from build123d import *

# Parameters (mm, degrees)
F0_R     = 4.7625
F1_DEPTH = 117.856
F2_W     = 9.525
F2_H     = 32.258
F3_DEPTH = 25.4
F4_DEPTH = 0.6985
F5_R     = 1.778
F6_DEPTH = 25.4
F8_DEPTH = 6.35
F9_SIZE  = 0.635


with BuildPart() as f1:
    # F0 (on Top) → F1 (new body)
    with BuildSketch(Plane.XY):
        Circle(F0_R)
    extrude(amount=F1_DEPTH)

    # F2 (on Right) → F3 (cut)
    with BuildSketch(Plane.YZ):
        with Locations((0, 29.337)):
            Rectangle(F2_W, F2_H)
    extrude(amount=F3_DEPTH, mode=Mode.SUBTRACT)

    # F2 (on Right) → F4 (cut)
    with BuildSketch(Plane.YZ):
        with Locations((0, 29.337)):
            Rectangle(F2_W, F2_H)
    extrude(amount=-F4_DEPTH, mode=Mode.SUBTRACT)

    # F5 (on face) → F6 (cut)
    with BuildSketch(Plane.YZ):
        with Locations((0, 39.6748)):
            Circle(F5_R)
        with Locations((0, 18.9738)):
            Circle(F5_R)
    extrude(amount=-F6_DEPTH, mode=Mode.SUBTRACT)

    # F7 (on face) → F8 (join)
    with BuildSketch(Plane.XY):
        with BuildLine():
            Line((3.928686, -2.691995), (3.928686, 2.691995))
            ThreePointArc((3.928686, 2.691995), (-4.7625, 0), (3.928686, -2.691995))
        make_face()
    extrude(amount=-F8_DEPTH)

    # F9
    f9_edges = [f1.edges().sort_by_distance(p)[0] for p in [
        (-4.7625, 0, 117.856),
    ]]
    chamfer(f9_edges, length=F9_SIZE)


solid = f1.part
Geometry: final body of the model. Coordinates: model frame, mm. A direction names the side the tool comes from. Give positions to 0.01 mm unless a question says otherwise; leave off trailing zeros. Write each loop counter-clockwise with the first axis right and the second up, starting at its lowest first coordinate (ties: lowest second). Pieces come first, ordered by that corner, then holes. Notation, with made-up numbers: (72, 79) - (110, 79) arc R27 cw to (110, 108) - close; hole circle Ø10 at (4, 36). An arc over 180 degrees is marked (long way). Return JSON: item names as keys, results as strings. Group by question number.
1) Set-up query: faces 3 (the flat face through (3.929, 0, -3)), 4 (the flat face through (-0.698, 0, 30)), 5 (the flat face through (0, 0, -6.35)). Return all of +Z, -Z, +X, -X, +Y, -Y with unobstructed straight access to the full face (end or side cutting, diameter ignored); none if empty.
2) Section B-B on z = 25.5. Return the cut outline in (x, y) (1 decimal).
3) Mould query, pull axis Y, two halves, no side actions, for faces 1 (the cylindrical face through (-2.703, -1.776, 39.753)), 2 (the flat face through (0, 0, 117.856)). Classes: released by +Y, released by -Y, zero draft, split by the parting line, or undercut.
4) Section A-A on y = 0. Return the cut outline in (x, z).
5) First-contact query: P1, Ø1, axis at y = -2.5, z = 94, coming from the -X side; P2, Ø5.5, axis at y = 0, z = 39.67, coming from the +X side; P3, Ø2, axis at y = -2, z = 39, coming from the -X side. Flat tips, straight axial feed; report the tip coordinate or a pass-through.
6) Section D-D on z = 103. Return the cut outline in (x, y) (1 decimal), plus the area to 3 significant figures.
7) Section C-C on x = -1.75. State how many separate pieces and enclosed holes the cut face has, plus the area to 3 significant figures.
8) Line query: line 1 (Z direction, x = -2.25, y = 0); line 2 (Z direction, x = 0, y = 2.75); line 3 (Y direction, x = -0.5, z = 91). Output: solid intervals per line, ascending.
Filled in:
{
 "1": {"face 3": "-Z, +X, +Y, -Y", "face 4": "+X, +Y, -Y", "face 5": "-Z, +X, -X, +Y, -Y"},
 "2": {"outline": "(-0.7, -4.7) - (-0.7, 4.7) arc R4.8 ccw to start"},
 "3": {"face 1": "undercut", "face 2": "zero draft"},
 "4": {"outline": "(-4.76, -6.35) - (3.93, -6.35) - (3.93, 0) - (4.76, 0) - (4.76, 13.21) - (-0.7, 13.21) - (-0.7, 17.2) - (-4.76, 17.2) - close; (-4.76, 20.75) - (-0.7, 20.75) - (-0.7, 37.9) - (-4.76, 37.9) - close; (-4.76, 41.45) - (-0.7, 41.45) - (-0.7, 45.47) - (4.76, 45.47) - (4.76, 117.22) - (4.13, 117.86) - (-4.13, 117.86) - (-4.76, 117.22) - close"},
 "5": {"P1": "stops at x = -4.32", "P2": "stops at x = -0.7", "P3": "stops at x = -4.6"},
 "6": {"outline": "circle Ø9.5 at (0, 0)", "area": "71.3 mm^2"},
 "7": {"separate pieces": "1", "enclosed holes": "2", "area": "1,080 mm^2"},
 "8": {"line 1": "z = -6.35 to 17.2, 20.75 to 37.9, 41.45 to 117.86", "line 2": "z = -6.35 to 13.21, 45.47 to 117.86", "line 3": "y = -4.74 to 4.74"}
}
